Source: three-view drawing plus pictorial views. Frame: mm from the lowest corner of the part. A direction names the side the tool comes from. Coordinates: 2 decimals unless noted, no trailing zeros. Order: outer loops, then holes, each group sorted by start corner. A loop starts at its lowest first (then second) coordinate and runs counter-clockwise, first axis right, second up. Notation, with made-up numbers: (89, 33.5) - (146, 33.5) arc R15 cw to (146, 45.5) - close; hole circle Ø1 at (27, 25.25). An arc over 180 degrees is marked (long way). One line per question, with ' | ' between items.
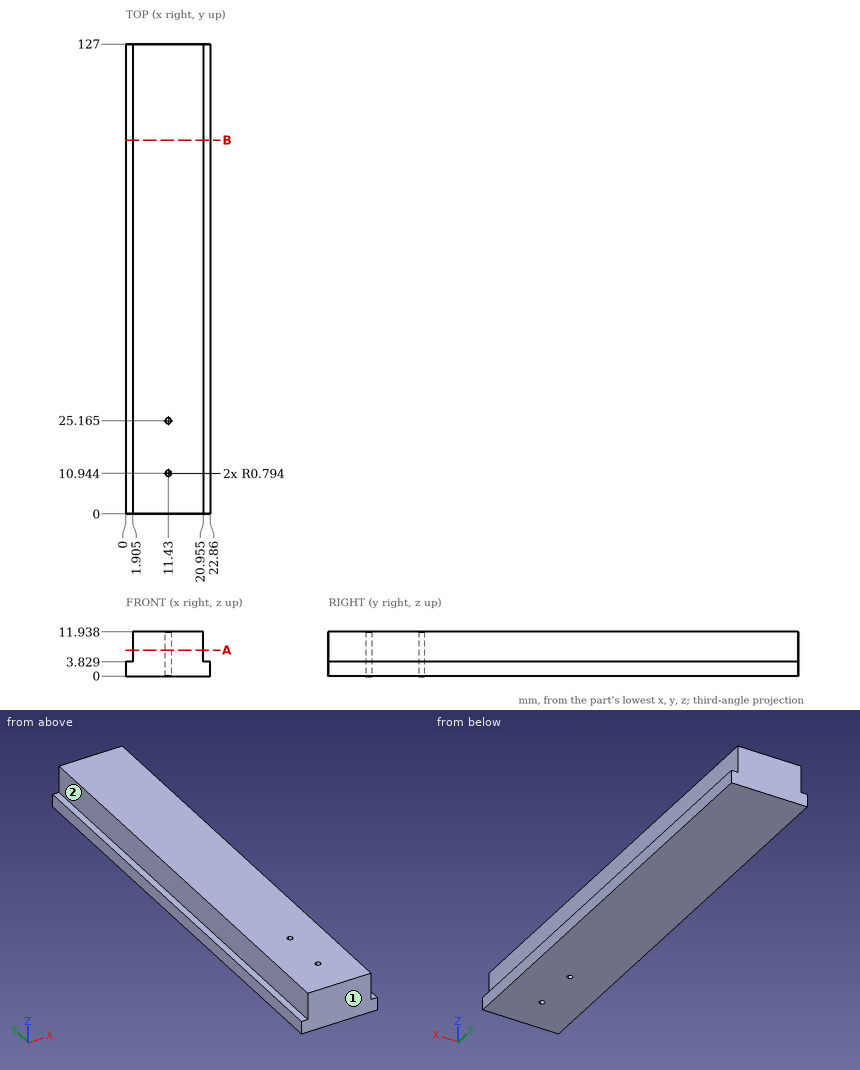
Item 1: Section B-B on y = 101. Return the cut outline in (x, z) (1 decimal), and give its area (3 significant figures).
Data:
outline: (0, 0) - (22.9, 0) - (22.9, 3.8) - (21, 3.8) - (21, 11.9) - (1.9, 11.9) - (1.9, 3.8) - (0, 3.8) - close | area: 242 mm^2
Item 2: Ray query, line 1 (X direction, y = 39, z = 8.25) (1 decimal); line 2 (X direction, y = 10.5, z = 9.75) (1 decimal); line 3 (Z direction, x = 21.25, y = 41). Return the intervals inside material, ascending.
Data:
line 1: 1.9 to 21 | line 2: 1.9 to 10.8, 12.1 to 21 | line 3: 0 to 3.83
Item 3: Section A-A on z = 7. Count the separate pieces of the cut face and the enclosed holes in it, and give its area (3 significant figures).
Data:
separate pieces: 1 | enclosed holes: 2 | area: 2,420 mm^2
Item 4: Contact query for flat-ended pins moving along their axis: P1, Ø5, axis at x = 16, y = 29, coming from the -Z side; P2, Ø4, axis at y = 50, z = 9.5, coming from the +X side (3 decimals); P3, Ø2, axis at y = 67.5, z = 9.5, coming from the -X side (3 decimals); P4, Ø1.5, axis at x = 22, y = 45.5, coming from the +Z side. Output: stop coordinate, or through.
Data:
P1: z = 0 | P2: x = 20.955 | P3: x = 1.905 | P4: z = 3.83
Item 5: Access query for the marked faces 1 and 2. Directions: +Z, -Z, +X, -X, +Y, -Y. A direction counts if a zero-diameter tool reaches every point of the face in a straight line with its end or side. Return the directions, or none.
Data:
face 1: +Z, -Z, +X, -X, -Y | face 2: +Z, -X, +Y, -Y
